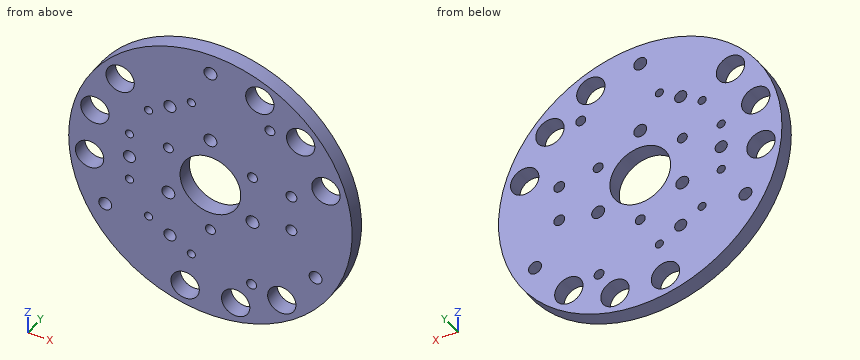
Autodesk Inventor part; units mm, degrees
ref_plane "YZ Plane" through (0, 0, 0) normal (1, 0, 0) x (0, 1, 0)
ref_plane "XZ Plane" through (0, 0, 0) normal (0, 1, 0) x (-1, 0, 0)
ref_plane "XY Plane" through (0, 0, 0) normal (0, 0, 1) x (1, 0, 0)
sketch "Sketch1" plane through (0, 0, 0) normal (0, 1, 0) x (-1, 0, 0)
  circle A0 centre (0, 0) radius 35
  circle A1 centre (0, 0) radius 7.5
  dimension "d0" = 70
  dimension "d129" = 15
extrude "Extrusion1" add sketch "Sketch1" along normal blind 4
sketch "Sketch2" plane through (0, 4, 0) normal (0, 1, 0) x (1, 0, 0)
  circle A0 centre (0, 0) radius 30 construction
  point P0 (0, -30)
  point P1 (-25.9808, 15)
  point P2 (25.9808, 15)
  dimension "d130" = 60
  dimension "d131" = 120
  dimension "d132" = 120
hole "Hole1" at (-25.9808, 4, -15) at (25.9808, 4, -15) at (0, 4, 30) direction (0, -1, 0) diameter 3.2 end through all
sketch "Sketch15" plane through (0, 4, 0) normal (0, 1, 0) x (1, 0, 0)
  circle A0 centre (0, 0) radius 30 construction
  circle A1 centre (0, -30) radius 1.6
  line L0 (0, 0) -> (0, -30) construction
  point P0 (12.2021, -27.4064)
  point P1 (0, -15)
  point P2 (17.6336, 24.2705)
  point P3 (-29.8357, 3.1359)
  point P4 (-22.2943, -20.0739)
  point P5 (28.5317, -9.2705)
  point P6 (-6.2374, 29.3444)
  dimension "d137" = 60
  dimension "d138" = 24
  dimension "d141" = 360
  dimension "d143" = 48
  dimension "d146" = 360
hole "Hole13" at (12.2021, 4, 27.4064) at (17.6336, 4, -24.2705) at (-29.8357, 4, -3.1359) at (-22.2943, 4, 20.0739) at (28.5317, 4, 9.2705) at (-6.2374, 4, -29.3444) direction (0, -1, 0) diameter 7 end through all
sketch "Sketch16" plane through (0, 4, 0) normal (0, 1, 0) x (1, 0, 0)
  circle A0 centre (0, 0) radius 12 construction
  point P0 (0, -12)
  point P1 (-10.3923, 6)
  point P2 (10.3923, 6)
  dimension "d155" = 24
  dimension "d156" = 120
  dimension "d157" = 120
hole "Hole14" at (0, 4, 12) at (-10.3923, 4, -6) at (10.3923, 4, -6) direction (0, -1, 0) diameter 3.2 end through all
sketch "Sketch17" plane through (0, 4, 0) normal (0, 1, 0) x (1, 0, 0)
  circle A0 centre (0, 0) radius 12 construction
  point P0 (0, 12)
  point P1 (-10.3923, -6)
  point P2 (10.3923, -6)
  dimension "d165" = 24
  dimension "d166" = 120
  dimension "d167" = 120
hole "Hole15" at (0, 4, -12) at (-10.3923, 4, 6) at (10.3923, 4, 6) direction (0, -1, 0) diameter 2.459 end through all
sketch "Sketch18" plane through (0, 4, 0) normal (0, 1, 0) x (1, 0, 0)
  point P0 (0, 0)
  point P1 (20, 4.5)
  point P2 (20, -4.5)
  dimension "d175" = 9
  dimension "d176" = 4.5
  dimension "d177" = 20
hole "Hole16" at (20, 4, -4.5) at (20, 4, 4.5) direction (0, -1, 0) diameter 2.7 end through all
sketch "Sketch19" plane through (0, 4, 0) normal (0, 1, 0) x (1, 0, 0)
  circle A0 centre (0, 0) radius 20 construction
  point P0 (-20, 0)
  point P1 (-10, 17.3205)
  point P2 (-10, -17.3205)
  dimension "d185" = 40
  dimension "d186" = 60
  dimension "d187" = 60
hole "Hole17" at (-20, 4, 0) at (-10, 4, -17.3205) at (-10, 4, 17.3205) direction (0, -1, 0) diameter 3 end through all
sketch "Sketch20" plane through (0, 4, 0) normal (0, 1, 0) x (1, 0, 0)
  circle A0 centre (-20, 0) radius 1.5
  point P0 (0, 0)
  point P1 (-20, 6.1)
  point P2 (-20, -6.1)
  point P3 (-4.7172, -20.3705)
  point P4 (-15.2828, -14.2705)
  point P5 (-15.2828, 14.2705)
  point P6 (-4.7172, 20.3705)
  point P7 (0, 0)
  dimension "d195" = 12.2
  dimension "d196" = 6.1
  dimension "d199" = 60
  dimension "d203" = 60
hole "Hole18" at (-20, 4, -6.1) at (-20, 4, 6.1) at (-4.7172, 4, 20.3705) at (-15.2828, 4, 14.2705) at (-15.2828, 4, -14.2705) at (-4.7172, 4, -20.3705) direction (0, -1, 0) diameter 2.013 end through all
sketch "Sketch21" plane through (0, 4, 0) normal (0, 1, 0) x (1, 0, 0)
  circle A0 centre (0, 0) radius 25 construction
  circle A1 centre (0, -30) radius 1.6
  point P0 (14.6946, -20.2254)
  point P1 (10.1684, 22.8386)
  dimension "d212" = 50
  dimension "d222" = 120
  dimension "d223" = 36
hole "Hole19" at (14.6946, 4, 20.2254) at (10.1684, 4, -22.8386) direction (0, -1, 0) diameter 2.459 end through all
sketch "Sketch22" plane through (0, 4, 0) normal (0, 1, 0) x (1, 0, 0)
  circle A0 centre (28.5317, -9.2705) radius 3.5
  line L0 (0, 0) -> (28.5317, -9.2705) construction
  circle A1 centre (12.2021, -27.4064) radius 3.5
  line L1 (0, 0) -> (12.2021, -27.4064) construction
  circle A2 centre (0, 0) radius 30 construction
  line L2 (0, 0) -> (22.2943, -20.0739) construction
  dimension "d224" = 48
  dimension "d227" = 24
hole "Hole20" at (22.2943, 4, 20.0739) direction (0, -1, 0) diameter 7 end through all
pattern_circular "Circular Pattern5" count 3 over 360 about axis through (0, 0, 0) along (0, 1, 0) of "Hole20"
equation "\"d227\" = 0.5 * d224"
properties part number "TopRing-2023-1" material "Copper"
CAD build for the part. Positions are in the model's coordinates, mm. Round coordinates to 2 decimals unless told otherwise and drop trailing zeros. Write each loop counter-clockwise with the first axis right and the second up, starting at its lowest first coordinate (ties: lowest second). Pieces come first, ordered by that corner, then holes. Notation, with made-up numbers: (70.25, 56.25) - (99.25, 56.25) arc R22 ccw to (99.25, 85.25) - close; hole circle Ø11 at (50.5, -31.75). An arc over 180 degrees is marked (long way). Return JSON: item names as keys, results as strings. Group by question number.
Item 1: Band-saw the part on A-A on x = 0. List the corners of the cut face in (y, z), plus the area to 3 significant figures.
Item 2: Band-saw the part on B-B on z = 29.5. List the corners of the cut face in (x, y), plus the area to 3 significant figures.
Item 3: Flat gauge pins, fed straight in: pin 1 Ø2 at (y, z) = (2.5, -9) entering from -X; pin 2 Ø1.2 at (x, z) = (-4.72, -20.37) entering from +Y (3 decimals); pin 3 Ø1 at (x, y) = (6, 1.5) entering from -Z. Where does each tip first touch, or does it go through?
Item 4: Probe probe 1 along Z at (x, y) = (0, 3.1); probe 2 along X at (y, z) = (2.1, 10); probe 3 along Z at (x, y) = (-15, 0.6). List the from-to ranges inside material, lowest first.
Item 5: Band-saw the part on C-C on y = 0.8. State how many separate pieces and enclosed holes the cut face has, plus the area to 3 significant figures.
Resolved:
{
 "1": {"outline": "(0, -35) - (4, -35) - (4, -13.23) - (0, -13.23) - close; (0, -10.77) - (4, -10.77) - (4, -7.5) - (0, -7.5) - close; (0, 7.5) - (4, 7.5) - (4, 10.4) - (0, 10.4) - close; (0, 13.6) - (4, 13.6) - (4, 28.4) - (0, 28.4) - close; (0, 31.6) - (4, 31.6) - (4, 35) - (0, 35) - close", "area": "185 mm²"},
 "2": {"outline": "(-18.83, 0) - (-1.52, 0) - (-1.52, 4) - (-18.83, 4) - close; (1.52, 0) - (9.4, 0) - (9.4, 4) - (1.52, 4) - close; (15.01, 0) - (18.83, 0) - (18.83, 4) - (15.01, 4) - close", "area": "116 mm²"},
 "3": {"pin 1": "stops at x = -34.07", "pin 2": "passes through", "pin 3": "stops at z = -34.57"},
 "4": {"probe 1": "z = -35 to -13.23, -10.77 to -7.5, 7.5 to 10.4, 13.6 to 28.4, 31.6 to 35", "probe 2": "x = -33.54 to -31.95, -25.11 to 25.11, 31.95 to 33.54", "probe 3": "z = -31.62 to -15.24, -13.3 to 13.3, 15.24 to 31.62"},
 "5": {"separate pieces": "1", "enclosed holes": "32", "area": "3,200 mm²"}
}
